```python
from build123d import *


with BuildPart() as f1:
    # F0 (on Front) → F1 (revolve)
    with BuildSketch(Plane.XZ):
        with BuildLine():
            Line((19.363788, 27.316456), (13.302453, 34.937789))
            ThreePointArc((13.302453, 34.937789), (8.135951, 32.884255), (3.914775, 29.266049))
            Line((3.914775, 29.266049), (3.948856, 7.517579))
            ThreePointArc((3.948856, 7.517579), (19.070867, 1.646298), (32.175929, 11.206869))
            Line((32.175929, 11.206869), (26.445522, 18.412104))
            Line((26.445522, 18.412104), (16.87957, 18.412104))
            Line((16.87957, 18.412104), (19.363788, 27.316456))
        make_face()
    revolve(axis=Axis((-0.029552, 0, 18.85881), (-0.001567, 0, 0.999999)))


solid = f1.part
```
Geometry: final body of the model. Coordinates: model frame, mm. A direction names the side the tool comes from. Coordinates: 2 decimals unless noted, no trailing zeros. Put each result on its own line as item: value.
(1) Access query for faces 3 (the face through (-13.815, -10.571, 18.363)), 4 (the face through (-3.511, 26.524, 18.015)). Directions: +Z, -Z, +X, -X, +Y, -Y. A direction counts if a zero-diameter tool reaches every point of the face in a straight line with its end or side. Return the directions, or none.
Answer sheet:
face 3: none
face 4: +Z
(2) Draft query along Y for faces 1 (the face through (-0.544, 3.927, 18.233)), 2 (the face through (-3.73, -16.66, 18.94)). Return one class per face: pulls with the +Y half, pulls with the -Y half, needs draft (parallel to the pull), parting line crosses it, or undercut.
Answer sheet:
face 1: undercut
face 2: parting line crosses it
(3) First-contact query: pin 1 (10 mm diameter, centred on y = 11, z = 7.5, fed in from +X); pin 2 (1.5 mm diameter, centred on y = 11.5, z = 28.5, fed in from +X); pin 3 (8 mm diameter, centred on x = 4, y = 10.5, fed in from +Z); pin 4 (1.5 mm diameter, centred on x = -25, y = -22, fed in from -Z). Flat tips, straight axial feed; report the tip coordinate or a pass-through.
Answer sheet:
pin 1: stops at x = 31.26
pin 2: stops at x = 15.34
pin 3: stops at z = 34.93
pin 4: passes through
(4) Material intervals for probe 1 along Y at (x, z) = (12.5, 7); probe 2 along Y at (x, z) = (-6, 6); probe 3 along Z at (x, y) = (-8.5, -20.5), sorted ascending.
Answer sheet:
probe 1: y = -26.6 to 26.6
probe 2: y = -27.79 to 27.79
probe 3: z = 2.31 to 18.36
